Input: part model. Units: mm. Frame: model coordinates. A direction names the side the tool comes from. Round coordinates to 2 decimals unless told otherwise and drop trailing zeros. Order: outer loops, then holes, each group sorted by start corner. A loop starts at its lowest first (then second) coordinate and runs counter-clockwise, first axis right, second up. Notation, with made-up numbers: (44.5, -3) -> (57.5, -3) arc R20 cw to (57.5, 26) -> close; hole circle Ø2 at (20.5, 86). An arc over 180 degrees is marked (long way). Use a Markdown table: item, result.
from build123d import *

# Parameters (mm, degrees)
BOSS_EXTRUDE1_DEPTH = 457.2
CUT_EXTRUDE1_DEPTH  = 458.772904943
SKETCH3_R           = 3.175
CUT_EXTRUDE2_DEPTH  = 458.772904943
SKETCH4_R           = 4.445
CUT_EXTRUDE3_DEPTH  = 406.4


with BuildPart() as part:
    # Sketch1 → Boss-Extrude1 (new body)
    with BuildSketch(Plane.XY):
        Polygon((5.08, 0), (1.905, -3.175), (10.795, -3.175), (7.62, 0), (12.7, 0), (12.7, -19.05), (0, -19.05), (0, 0), align=None)
    extrude(amount=BOSS_EXTRUDE1_DEPTH)

    # Sketch2 → Cut-Extrude1 (cut, through all)
    with BuildSketch(Plane(origin=(12.7, 0, 0), x_dir=(0, 0, -1), z_dir=(1, 0, 0))):
        with BuildLine():
            Line((-457.2, 0), (-457.2, -19.05))
            Line((-457.2, -19.05), (-438.15, -19.05))
            ThreePointArc((-438.15, -19.05), (-451.620384182, -13.470384182), (-457.2, 0))
        make_face()
    extrude(amount=-CUT_EXTRUDE1_DEPTH, mode=Mode.SUBTRACT)

    # Sketch3 → Cut-Extrude2 (cut, through all)
    with BuildSketch(Plane(origin=(12.7, 0, 0), x_dir=(0, 0, -1), z_dir=(1, 0, 0))):
        with Locations(Location((-444.885192091, -6.735192091, 0), (0, 0, 90))):
            Circle(SKETCH3_R)
    extrude(amount=-CUT_EXTRUDE2_DEPTH, mode=Mode.SUBTRACT)

    # Sketch4 → Cut-Extrude3 (cut)
    with BuildSketch(Plane(origin=(0, 0, 0), x_dir=(-1, 0, 0), z_dir=(0, 0, -1))):
        with Locations((-6.35, -11.43)):
            Circle(SKETCH4_R)
    extrude(amount=-CUT_EXTRUDE3_DEPTH, mode=Mode.SUBTRACT)


solid = part.part
1) Cut plane A-A on z = 300. Return loops of the section in (x, y) (3 decimals), and give its area (3 significant figures).
Results found:
| item | result |
|---|---|
| outline | (0, -19.05) -> (12.7, -19.05) -> (12.7, 0) -> (7.62, 0) -> (10.795, -3.175) -> (1.905, -3.175) -> (5.08, 0) -> (0, 0) -> close; hole circle Ø8.89 at (6.35, -11.43) |
| area | 162 mm² |
2) Pin query (flat end, axial travel): pin 1 Ø4 at (y, z) = (-6.74, 444.89) entering from +X; pin 2 Ø5.5 at (x, y) = (6.35, -11.43) entering from -Z. Return the tip coordinate at first contact, or that it passes through.
Results found:
| item | result |
|---|---|
| pin 1 | passes through |
| pin 2 | stops at z = 406.4 |
3) Line query: L1, parallel to X at y = -11.75, z = 277.5; L2, parallel to Y at x = 4, z = 324 (3 decimals); L3, parallel to Y at x = 9.75, z = 320 (3 decimals). Output: solid intervals per line, ascending. Write a range as [from, to].
Results found:
| item | result |
|---|---|
| L1 | x = [0, 1.92], [10.78, 12.7] |
| L2 | y = [-19.05, -15.203], [-7.657, -3.175], [-1.08, 0] |
| L3 | y = [-19.05, -14.293], [-8.567, -3.175], [-2.13, 0] |
4) Set-up query: faces 1 (the cylindrical face through (6.44, -13.62, 451.47)), 2 (the flat face through (6, -11, 406.4)). Return all of +Z, -Z, +X, -X, +Y, -Y with unobstructed straight access to the full face (end or side cutting, diameter ignored); none if empty.
Results found:
| item | result |
|---|---|
| face 1 | +Z, +X, -X, -Y |
| face 2 | -Z |
5) Pull-direction query (Y, two-part tool) for faces 3 (the cylindrical face through (7.31, -15.77, 200.36)), 4 (the flat face through (9, -7, 0)), 5 (the flat face through (6, -19.05, 216)); classes: +Y half, -Y half, draft (parallel to the pull), parting line (faces both ways), or undercut.
Results found:
| item | result |
|---|---|
| face 3 | undercut |
| face 4 | draft |
| face 5 | -Y half |
